Source: CAD feature listing. Evaluate the final solid. Frame: model axes, mm. A direction names the side the tool comes from. Give positions to 0.01 mm unless a question says otherwise; leave off trailing zeros. Write each loop counter-clockwise with the first axis right and the second up, starting at its lowest first coordinate (ties: lowest second). Pieces come first, ordered by that corner, then holes. Notation, with made-up numbers: (38.25, -10.5) -> (59.25, -10.5) arc R28 cw to (59.25, 24.5) -> close; hole circle Ø7 at (49, -35.75). An arc over 180 degrees is marked (long way). Write item = value, one per line.
from build123d import *

# Parameters (mm, degrees)
SKETCH1_R                = 35
BOSS_EXTRUDE1_DEPTH      = 25
SHELL1_T                 = -3
FILLET1_R                = 10
BOSS_EXTRUDE2_START      = -5
SKETCH4_R                = 4
BOSS_EXTRUDE2_DEPTH      = 5
CIRPATTERN1_COUNT        = 3
CUT_EXTRUDE1_DEPTH       = 72.991907702
BOSS_EXTRUDE3_DEPTH      = 5
BOSS_EXTRUDE3_DEPTH_BACK = 3
SKETCH7_R                = 12.5
FILLET2_R                = 2
SKETCH8_R                = 7.5
CUT_EXTRUDE2_DEPTH       = 74.877160033


with BuildPart() as part:
    # Sketch1 → Boss-Extrude1 (new body)
    with BuildSketch(Plane(origin=(0, 0, 0), x_dir=(1, 0, 0), z_dir=(0, 1, 0))):
        with Locations(Location((0, 0, 0), (0, 0, 270))):
            Circle(SKETCH1_R)
    extrude(amount=BOSS_EXTRUDE1_DEPTH)

    # Shell1
    shell1_openings = [part.faces().sort_by_distance(p)[0] for p in [
        (0, 25, 0),
    ]]
    offset(amount=SHELL1_T, openings=shell1_openings, kind=Kind.INTERSECTION)

    # Fillet1
    fillet1_edges = [part.edges().sort_by_distance(p)[0] for p in [
        (0, 0, -35),
    ]]
    fillet(fillet1_edges, radius=FILLET1_R)

    # Sketch4 → Boss-Extrude2 (add)
    with BuildSketch(Plane(origin=(0, 25, 0), x_dir=(1, 0, 0), z_dir=(0, 1, 0)).offset(BOSS_EXTRUDE2_START)):
        with BuildLine():
            Line((-8, 42.5), (-8, 34.073450075))
            ThreePointArc((-8, 34.073450075), (0, 35), (8, 34.073450075))
            Line((8, 34.073450075), (8, 42.5))
            ThreePointArc((8, 42.5), (0, 50.5), (-8, 42.5))
        make_face()
        with Locations(Location((0, 42.5, 0), (0, 0, 270))):
            Circle(SKETCH4_R, mode=Mode.SUBTRACT)
    boss_extrude2 = extrude(amount=BOSS_EXTRUDE2_DEPTH)

    # CirPattern1: Boss-Extrude2 ×3 about axis
    cirpattern1_axis = Axis((0, 0, 0), (0, 1, 0))
    for i in range(1, CIRPATTERN1_COUNT):
        add(boss_extrude2.rotate(cirpattern1_axis, i * 360 / CIRPATTERN1_COUNT))

    # Sketch5 → Cut-Extrude1 (cut, through all)
    with BuildSketch(Plane.XZ):
        with BuildLine():
            Line((-16, 20), (-16, -20))
            ThreePointArc((-16, -20), (-18, -22), (-20, -20))
            Line((-20, -20), (-20, 20))
            ThreePointArc((-20, 20), (-18, 22), (-16, 20))
        make_face()
        with BuildLine():
            Line((-10, 20), (-10, -20))
            ThreePointArc((-10, -20), (-12, -22), (-14, -20))
            Line((-14, -20), (-14, 20))
            ThreePointArc((-14, 20), (-12, 22), (-10, 20))
        make_face()
        with BuildLine():
            Line((-4, 20), (-4, -20))
            ThreePointArc((-4, -20), (-6, -22), (-8, -20))
            Line((-8, -20), (-8, 20))
            ThreePointArc((-8, 20), (-6, 22), (-4, 20))
        make_face()
        with BuildLine():
            Line((2, 20), (2, -20))
            ThreePointArc((2, -20), (0, -22), (-2, -20))
            Line((-2, -20), (-2, 20))
            ThreePointArc((-2, 20), (0, 22), (2, 20))
        make_face()
        with BuildLine():
            Line((8, 20), (8, -20))
            ThreePointArc((8, -20), (6, -22), (4, -20))
            Line((4, -20), (4, 20))
            ThreePointArc((4, 20), (6, 22), (8, 20))
        make_face()
        with BuildLine():
            Line((14, 20), (14, -20))
            ThreePointArc((14, -20), (12, -22), (10, -20))
            Line((10, -20), (10, 20))
            ThreePointArc((10, 20), (12, 22), (14, 20))
        make_face()
        with BuildLine():
            Line((20, 20), (20, -20))
            ThreePointArc((20, -20), (18, -22), (16, -20))
            Line((16, -20), (16, 20))
            ThreePointArc((16, 20), (18, 22), (20, 20))
        make_face()
    extrude(amount=-CUT_EXTRUDE1_DEPTH, mode=Mode.SUBTRACT)

    # Sketch7 → Boss-Extrude3 (add, two sides: drawn at the far end of the back side and taken through both)
    with BuildSketch(Plane.XZ.offset(-BOSS_EXTRUDE3_DEPTH_BACK)):
        with Locations(Location((0, 0, 0), (0, 0, 270))):
            Circle(SKETCH7_R)
    extrude(amount=BOSS_EXTRUDE3_DEPTH + BOSS_EXTRUDE3_DEPTH_BACK)

    # Fillet2
    fillet2_edges = [part.edges().sort_by_distance(p)[0] for p in [
        (0, -5, 12.5),
    ]]
    fillet(fillet2_edges, radius=FILLET2_R)

    # Sketch8 → Cut-Extrude2 (cut, through all)
    with BuildSketch(Plane.XZ.offset(5)):
        with Locations(Location((0, 0, 0), (0, 0, 270))):
            Circle(SKETCH8_R)
    extrude(amount=-CUT_EXTRUDE2_DEPTH, mode=Mode.SUBTRACT)


solid = part.part
1) Material intervals for L1, parallel to X at y = 21.6, z = -42.5; L2, parallel to X at y = -2.5, z = 0; L3, parallel to Y at x = -5.5, z = -7, sorted ascending.
Computed:
L1 = -8 to -4, 4 to 8
L2 = -12.5 to -7.5, 7.5 to 12.5
L3 = -5 to 3
2) Draft query along Z for faces 1 (the cylindrical face through (36.982, 22.465, 17.254)), 2 (the flat face through (30, 25, -14)), 3 (the flat face through (29.106, 22.465, 26.042)). Return one class per face: pulls with the +Z half, pulls with the -Z half, needs draft (parallel to the pull), parting line crosses it, or undercut.
Computed:
face_1 = undercut
face_2 = needs draft
face_3 = pulls with the +Z half
3) Contact query for flat-ended pins moving along their axis: pin 1 (4 mm diameter, centred on x = 18, y = 7, fed in from -Z); pin 2 (17.5 mm diameter, centred on x = -4, z = -42, fed in from -Y); pin 3 (1 mm diameter, centred on y = 11, z = 8, fed in from -X); pin 4 (5 mm diameter, centred on x = 5.5, z = -1, fed in from -Y). Output: stop coordinate, or through.
Computed:
pin_1 = -30.77
pin_2 = 4.64
pin_3 = -34.19
pin_4 = -5
4) Cut plane A-A (x = 36.5). Return the cut outline in (y, z).
Computed:
outline = (20, 11.84) -> (25, 11.84) -> (25, 17.26) -> (20, 17.26) -> close; (20, 25.24) -> (25, 25.24) -> (25, 29.24) -> (20, 29.24) -> close
5) Access query for faces 4 (the cylindrical face through (-31.24, 13.85, -6.94)), 5 (the cylindrical face through (-34.168, 17.395, -7.587)), 6 (the flat face through (-34, 20, 18)), 7 (the flat face through (-10, 1, 14)). Directions: +Z, -Z, +X, -X, +Y, -Y. A direction counts if a zero-diameter tool reaches every point of the face in a straight line with its end or side. Return the directions, or none.
Computed:
face_4 = +Y
face_5 = -Y
face_6 = +Z, -X, -Y
face_7 = +Y, -Y
6) Cut plane B-B (y = 14.75). Return the cut outline in (x, z), then the cut area to 3 significant figures.
Computed:
outline = circle Ø70 at (0, 0); hole circle Ø64 at (0, 0)
area = 631 mm²
7) Cut plane C-C (z = -18). State how many separate pieces and enclosed holes the cut face has, then the cut area to 3 significant figures.
Computed:
separate_pieces = 8
enclosed_holes = 0
area = 201 mm²
